from build123d import *

# Parameters (mm, degrees)
F1_DEPTH = 114.3
F2_DEPTH = 25.4
F3_R     = 25.4


with BuildPart() as f1:
    # F0 (on Top) → F1 (new body)
    with BuildSketch(Plane.XY):
        Polygon((457.2, 0), (-457.2, 0), (-457.2, -508), (-431.8, -508), (-254, -508), (-254, -311.15), (254, -311.15), (254, -508), (431.8, -508), (457.2, -508), align=None)
    extrude(amount=F1_DEPTH)

    # F0 (on Top) → F2 (join)
    with BuildSketch(Plane.XY):
        Polygon((-254, -508), (-431.8, -508), (-431.8, -755.65), (431.8, -755.65), (431.8, -508), (254, -508), (254, -311.15), (-254, -311.15), align=None)
    extrude(amount=F2_DEPTH)

    # F3
    f3_edges = [f1.edges().sort_by_distance(p)[0] for p in [
        (-457.2, -508, 57.15),
        (-431.8, -755.65, 12.7),
        (-254, -508, 69.85),
        (254, -311.15, 69.85),
        (254, -508, 69.85),
        (457.2, -508, 57.15),
        (431.8, -755.65, 12.7),
        (-254, -311.15, 69.85),
        (457.2, 0, 57.15),
        (-457.2, 0, 57.15),
    ]]
    fillet(f3_edges, radius=F3_R)


solid = f1.part
Here's how the part is built. I have some questions about the finished solid (model axes, mm). A direction names the side the tool comes from. Coordinates: 2 decimals unless noted, no trailing zeros. Write each loop counter-clockwise with the first axis right and the second up, starting at its lowest first coordinate (ties: lowest second). Pieces come first, ordered by that corner, then holes. Notation, with made-up numbers: (1.25, 62) - (13.25, 62) arc R23 cw to (13.25, 82) - close; hole circle Ø5 at (44, 29.25). An arc over 180 degrees is marked (long way). Use one line per item in the form item = value.
1) I need wall thicknesses on line 1 (Y direction, x = 50, z = 36.5); line 2 (X direction, y = -343, z = 104); line 3 (Z direction, x = -166, y = -378). Which ranges of each line are inside material? Lowest first, please.
Solved:
line_1 = -311.15 to 0
line_2 = -457.2 to -254, 254 to 457.2
line_3 = 0 to 25.4
2) Suppose I cut it at C-C, the plane x = -306. Write out the boundary of the cut face in (y, z).
Solved:
outline = (-755.65, 0) - (0, 0) - (0, 114.3) - (-508, 114.3) - (-508, 25.4) - (-755.65, 25.4) - close
3) Thinking about a two-plate mould opening in X: for faces 4 (the flat face through (-457.2, -251, 56)), 5 (the flat face through (457.2, -257, 56)), 6 (the cylindrical face through (246.76, -318.79, 70.47)), which applies, released by +X, released by -X, zero draft, split by the parting line, or undercut?
Solved:
face_4 = released by -X
face_5 = released by +X
face_6 = undercut
4) I'm going to push flat-ended pins straight in: P1, Ø1.5, axis at x = -102.5, y = -385, coming from the +Z side; P2, Ø12.5, axis at y = -608, z = 13, coming from the +X side; P3, Ø1.5, axis at y = -496, z = 93, coming from the +X side. Where does each tip first touch, or does it pass through?
Solved:
P1 = 25.4
P2 = 431.8
P3 = 453.83
5) Suppose I cut it at B-B, the plane z = 38. Write out the boundary of the cut face in (x, y).
Solved:
outline = (-457.2, -482.6) arc R25.4 ccw to (-431.8, -508) - (-279.4, -508) arc R25.4 ccw to (-254, -482.6) - (-254, -336.55) arc R25.4 cw to (-228.6, -311.15) - (228.6, -311.15) arc R25.4 cw to (254, -336.55) - (254, -482.6) arc R25.4 ccw to (279.4, -508) - (431.8, -508) arc R25.4 ccw to (457.2, -482.6) - (457.2, -25.4) arc R25.4 ccw to (431.8, 0) - (-431.8, 0) arc R25.4 ccw to (-457.2, -25.4) - close
6) Suppose I cut it at A-A, the plane x = 38.5. Write out the boundary of the cut face in (y, z), plus the area to 3 significant figures.
Solved:
outline = (-755.65, 0) - (0, 0) - (0, 114.3) - (-311.15, 114.3) - (-311.15, 25.4) - (-755.65, 25.4) - close
area = 46,900 mm2
7) On a 3-axis mill with a long thin cutter (end or side, diameter ignored), from which of +Z, -Z, +X, -X, +Y, -Y can I reach the whole of each face in a straight line? I mean faces 1 (the flat face through (254, -409, 69)), 2 (the flat face through (-431.8, -618, 13)), 3 (the flat face through (-357, -508, 69)). Say none if no direction works.
Solved:
face_1 = +Z, -Y
face_2 = +Z, -Z, -X, -Y
face_3 = +Z, +X, -X, -Y
